```python
from build123d import *

# Parameters (mm, degrees)
SKETCH1_W           = 6.35
SKETCH1_H           = 6.35
BOSS_EXTRUDE1_DEPTH = 1.27
SKETCH2_W           = 6.35
SKETCH2_H           = 1.143
BOSS_EXTRUDE2_DEPTH = 10.16
CUT_EXTRUDE1_REACH  = 3.143
SKETCH4_R           = 1.397


with BuildPart() as part:
    # Sketch1 → Boss-Extrude1 (new body)
    with BuildSketch(Plane(origin=(0, 0, 0), x_dir=(1, 0, 0), z_dir=(0, 1, 0))):
        Rectangle(SKETCH1_W, SKETCH1_H)
    extrude(amount=BOSS_EXTRUDE1_DEPTH)

    # Sketch2 → Boss-Extrude2 (add)
    with BuildSketch(Plane(origin=(0, 1.27, 0), x_dir=(1, 0, 0), z_dir=(0, 1, 0))):
        with Locations((0, 2.6035)):
            Rectangle(SKETCH2_W, SKETCH2_H)
    extrude(amount=BOSS_EXTRUDE2_DEPTH)

    # Sketch4 → Cut-Extrude1 (cut, up to next)
    with BuildSketch(Plane.XY.offset(-2.032), mode=Mode.PRIVATE) as cut_extrude1_sk1:
        with Locations((0, 3.048)):
            Circle(SKETCH4_R)
    cut_extrude1_tool1 = extrude(cut_extrude1_sk1.sketch, amount=-CUT_EXTRUDE1_REACH, mode=Mode.PRIVATE) & part.part
    add(cut_extrude1_tool1.solids().sort_by_distance((0, 3.048, -2.032))[0], mode=Mode.SUBTRACT)


solid = part.part
```
The model under review builds one solid part; all positions refer to its coordinate system, in mm. A direction names the side the tool comes from. Give positions to 0.01 mm unless a question says otherwise; leave off trailing zeros. Loops run counter-clockwise (first coordinate to the right, second up) from the corner with the lowest first, then second, coordinate; pieces in that order, holes last. Notation, with made-up numbers: (83, 64) - (133, 64) arc R13 ccw to (133, 81) - close; hole circle Ø1 at (54.25, -39.75). An arc over 180 degrees is marked (long way). Answer as a JSON object with one key per item and string values.
Q1. Add section C-C on x = 2.5. State the section outline as (y, z) points (3 decimals), plus the area to 3 significant figures.
Worked out:
{"outline": "(0, -3.175) - (11.43, -3.175) - (11.43, -2.032) - (1.27, -2.032) - (1.27, 3.175) - (0, 3.175) - close", "area": "19.7 mm^2"}
Q2. Add section D-D on z = -2.25. State the section outline as (x, y) points (3 decimals), plus the area to 3 significant figures.
Worked out:
{"outline": "(-3.175, 0) - (3.175, 0) - (3.175, 11.43) - (-3.175, 11.43) - close; hole circle Ø2.794 at (0, 3.048)", "area": "66.4 mm^2"}
Q3. Insertion check: pin 1 (1 mm diameter, centred on x = -2.5, z = -0.5, fed in from +Y). The pin has a flat end and moves straight along its axis. Give the tip position at first contact, or say it passes through.
Worked out:
{"pin 1": "stops at y = 1.27"}
Q4. Add section B-B on y = 2.25. State the section outline as (x, z) points (3 decimals), plus the area to 3 significant figures.
Worked out:
{"outline": "(-3.175, -3.175) - (-1.147, -3.175) - (-1.147, -2.032) - (-3.175, -2.032) - close; (1.147, -3.175) - (3.175, -3.175) - (3.175, -2.032) - (1.147, -2.032) - close", "area": "4.64 mm^2"}
Q5. Add section A-A on x = 0. State the section outline as (y, z) points (3 decimals), plus the area to 3 significant figures.
Worked out:
{"outline": "(0, -3.175) - (1.651, -3.175) - (1.651, -2.032) - (1.27, -2.032) - (1.27, 3.175) - (0, 3.175) - close; (4.445, -3.175) - (11.43, -3.175) - (11.43, -2.032) - (4.445, -2.032) - close", "area": "16.5 mm^2"}
Q6. Mouldability with a two-part tool opening along Y and no side actions: class faces 3 (the flat face through (-3.175, 4, -2.3)), 4 (the cylindrical face through (-0.303, 1.684, -2.595)), 5 (the flat face through (0, 0, 0)), 6 (the flat face through (0, 11.43, -3)) as +Y half, -Y half, draft (parallel to the pull), parting line (faces both ways), or undercut.
Worked out:
{"face 3": "draft", "face 4": "undercut", "face 5": "-Y half", "face 6": "+Y half"}
Q7. To check wall thickness, follow line 1 along Y through (x, z) = (0, -2.45) (3 decimals); line 2 along Z through (x, y) = (2.5, 8.75) (3 decimals); line 3 along Y through (x, z) = (-0.5, 0.5). State the ranges of each line that lie inside material, in increasing order.
Worked out:
{"line 1": "y = 0 to 1.651, 4.445 to 11.43", "line 2": "z = -3.175 to -2.032", "line 3": "y = 0 to 1.27"}
Q8. For faces 1 (the flat face through (0, 1.27, 1)), 2 (the flat face through (0, 6, -3.175)), list the 3-axis set-ups (+Z, -Z, +X, -X, +Y, -Y) from which the entire face can be reached by the end or side of a thin tool; tool diameter is ignored.
Worked out:
{"face 1": "+Z, +X, -X, +Y", "face 2": "-Z, +X, -X, +Y, -Y"}
